For this review, take the finished solid that the model builds, in its own axes (mm). A direction names the side the tool comes from. Coordinates: 2 decimals unless noted, no trailing zeros. Loops run counter-clockwise (first coordinate to the right, second up) from the corner with the lowest first, then second, coordinate; pieces in that order, holes last. Notation, with made-up numbers: M 49,41.25 L 89,41.25 A22 cw 89,74.25 Z; hole C 71.5,40.25 d5. An arc over 180 degrees is marked long. Use one line per item in the form item = value.
```python
from build123d import *

# Parameters (mm, degrees)
SKIZZE3_W                            = 46.7
SKIZZE3_H                            = 6
AUFSATZ_LINEAR_AUSTRAGEN1_DEPTH      = 12.65
AUFSATZ_LINEAR_AUSTRAGEN1_DEPTH_BACK = 12.65
SKIZZE4_OUTSIDE_W                    = 59.39
SKIZZE4_OUTSIDE_H                    = 37.99
SKIZZE4_OUTSIDE_W_2                  = 35.95
SKIZZE4_OUTSIDE_H_2                  = 21.7
SCHNITT_LINEAR_AUSTRAGEN1_DEPTH      = 237
SKIZZE7_R                            = 4.5
SKIZZE7_R_2                          = 1.5
SCHNITT_LINEAR_AUSTRAGEN2_DEPTH      = 237
SCHNITT_LINEAR_START                 = -10.85
THREADHOLESSIDE_R                    = 1.25
SCHNITT_LINEAR_AUSTRAGEN3_DEPTH      = 6
SCHNITT_LINEAR_START_2               = 10.85
THREADHOLESSIDE_2_R                  = 1.25
SCHNITT_LINEAR_AUSTRAGEN4_DEPTH      = 6


with BuildPart() as part:
    # Skizze3 → Aufsatz-Linear austragen1 (new body, two sides)
    with BuildSketch(Plane.XY) as aufsatz_linear_austragen1_sk:
        with Locations((0, 234)):
            Rectangle(SKIZZE3_W, SKIZZE3_H)
    extrude(amount=AUFSATZ_LINEAR_AUSTRAGEN1_DEPTH)
    extrude(aufsatz_linear_austragen1_sk.sketch, amount=-AUFSATZ_LINEAR_AUSTRAGEN1_DEPTH_BACK)

    # Skizze4 outside → Schnitt-Linear austragen1 (cut)
    with BuildSketch(Plane(origin=(0, 0, 0), x_dir=(1, 0, 0), z_dir=(0, 1, 0))):
        Rectangle(SKIZZE4_OUTSIDE_W, SKIZZE4_OUTSIDE_H)
        with Locations((5.375, 0)):
            Rectangle(SKIZZE4_OUTSIDE_W_2, SKIZZE4_OUTSIDE_H_2, mode=Mode.SUBTRACT)
    extrude(amount=SCHNITT_LINEAR_AUSTRAGEN1_DEPTH, mode=Mode.SUBTRACT)

    # Skizze7 → Schnitt-Linear austragen2 (cut)
    with BuildSketch(Plane(origin=(0, 0, 0), x_dir=(1, 0, 0), z_dir=(0, 1, 0))):
        Circle(SKIZZE7_R)
        with Locations((14, 0)):
            Circle(SKIZZE7_R_2)
    extrude(amount=SCHNITT_LINEAR_AUSTRAGEN2_DEPTH, mode=Mode.SUBTRACT)

    # ThreadHolesSide → Schnitt-Linear austragen3 (cut)
    with BuildSketch(Plane.XY.offset(SCHNITT_LINEAR_START)):
        with Locations((18.35, 234)):
            Circle(THREADHOLESSIDE_R)
        with Locations((-8, 234)):
            Circle(THREADHOLESSIDE_R)
    extrude(amount=SCHNITT_LINEAR_AUSTRAGEN3_DEPTH, mode=Mode.SUBTRACT)

    # ThreadHolesSide<2> → Schnitt-Linear austragen4 (cut)
    with BuildSketch(Plane.XY.offset(SCHNITT_LINEAR_START_2)):
        with Locations((18.35, 234)):
            Circle(THREADHOLESSIDE_2_R)
        with Locations((-8, 234)):
            Circle(THREADHOLESSIDE_2_R)
        with Locations((18.35, 615)):
            Circle(THREADHOLESSIDE_2_R)
        with Locations((-8, 615)):
            Circle(THREADHOLESSIDE_2_R)
    extrude(amount=-SCHNITT_LINEAR_AUSTRAGEN4_DEPTH, mode=Mode.SUBTRACT)


solid = part.part
```
1. Tool access review of faces 4 (the face through (18.08, 232.78, 7.89)), 5 (the face through (18, 234, -4.85)), 6 (the face through (5, 234, 10.85)): name each direction out of +Z, -Z, +X, -X, +Y, -Y from which nothing blocks a thin tool from reaching the whole face with its end or side.
Computed values:
face_4 = +Z
face_5 = -Z
face_6 = +Z, +X, -X, +Y, -Y
2. Consider section D-D on z = -3.25. Write out the cut boundary in (x, y), plus the area to 3 significant figures.
Computed values:
outline = M -12.6,231 L -3.11,231 L -3.11,237 L -12.6,237 Z; M 3.11,231 L 23.35,231 L 23.35,237 L 3.11,237 Z
area = 178 mm2
3. Draft analysis for pull direction Y (two halves, no side actions). For faces 1 (the face through (-8.27, 232.78, -7.89)), 2 (the face through (12.5, 233.96, -0.07)), 3 (the face through (5, 237, 0)), state which applies: +Y half, -Y half, draft (parallel to the pull), parting line (faces both ways), or undercut.
Computed values:
face_1 = undercut
face_2 = draft
face_3 = +Y half
4. Wall thickness on line 1 along X through (y, z) = (234, -7.15); line 2 along X through (y, z) = (232.6, 0); line 3 along Z through (x, y) = (14, 234): over which ranges is each line inside the solid? List them lowest first. Write a range as from..to.
Computed values:
line_1 = -12.6..-9.25, -6.75..17.1, 19.6..23.35
line_2 = -12.6..-4.5, 4.5..12.5, 15.5..23.35
line_3 = -10.85..-1.5, 1.5..10.85
5. For pin 1 Ø0.8 at (x, y) = (18.5, 234.5) entering from +Z; pin 2 Ø2 at (x, y) = (-7.5, 234.5) entering from -Z; pin 3 Ø2 at (x, y) = (-8, 234) entering from -Z, all flat-tipped, find the tip position at first contact; note any pin that passes through.
Computed values:
pin_1 = 4.85
pin_2 = -10.85
pin_3 = -4.85
6. Consider section C-C on y = 231.4. Write out the cut boundary in (x, z), plus the area to 3 significant figures.
Computed values:
outline = M -12.6,-10.85 L 23.35,-10.85 L 23.35,10.85 L -12.6,10.85 Z; hole C 0,0 d9; hole C 14,0 d3
area = 709 mm2
7. Consider section B-B on z = 0. Write out the cut boundary in (x, y).
Computed values:
outline = M -12.6,231 L -4.5,231 L -4.5,237 L -12.6,237 Z; M 4.5,231 L 12.5,231 L 12.5,237 L 4.5,237 Z; M 15.5,231 L 23.35,231 L 23.35,237 L 15.5,237 Z
8. Consider section A-A on x = 0. Write out the cut boundary in (y, z), plus the area to 3 significant figures.
Computed values:
outline = M 231,-10.85 L 237,-10.85 L 237,-4.5 L 231,-4.5 Z; M 231,4.5 L 237,4.5 L 237,10.85 L 231,10.85 Z
area = 76.2 mm2
